```python
from build123d import *

# Parameters (mm, degrees)
SKETCH1_W      = 16
SKETCH1_H      = 16
EXTRUDE1_DEPTH = 240
SKETCH2_W      = 13
SKETCH2_H      = 13
EXTRUDE2_DEPTH = 242.064306773
SKETCH3_R      = 4
SKETCH3_R_2    = 1.85
EXTRUDE3_DEPTH = 242.064306773
SKETCH4_R      = 4
SKETCH4_R_2    = 1.85
EXTRUDE4_DEPTH = 242.064306773
FILLET1_R      = 1


with BuildPart() as part:
    # Sketch1 → Extrude1 (new body)
    with BuildSketch(Plane.XY):
        with Locations((8, 8)):
            Rectangle(SKETCH1_W, SKETCH1_H)
    extrude(amount=-EXTRUDE1_DEPTH)

    # Sketch2 → Extrude2 (cut, through all)
    with BuildSketch(Plane.XY):
        with Locations((8, 8)):
            Rectangle(SKETCH2_W, SKETCH2_H)
    extrude(amount=-EXTRUDE2_DEPTH, mode=Mode.SUBTRACT)

    # Sketch3 → Extrude3 (cut, through all)
    with BuildSketch(Plane(origin=(0, 16, 0), x_dir=(1, 0, 0), z_dir=(0, 1, 0))):
        with Locations(Location((8, 64, 0), (0, 0, 270))):
            Circle(SKETCH3_R)
        with Locations(Location((8, 32, 0), (0, 0, 270))):
            Circle(SKETCH3_R)
        with Locations((8, 0)):
            Circle(SKETCH3_R)
        with Locations(Location((8, 96, 0), (0, 0, 270))):
            Circle(SKETCH3_R)
        with Locations(Location((8, 128, 0), (0, 0, 270))):
            Circle(SKETCH3_R)
        with Locations(Location((8, 160, 0), (0, 0, 270))):
            Circle(SKETCH3_R)
        with Locations(Location((8, 192, 0), (0, 0, 270))):
            Circle(SKETCH3_R)
        with Locations(Location((8, 224, 0), (0, 0, 270))):
            Circle(SKETCH3_R)
        with Locations((8, 256)):
            Circle(SKETCH3_R)
        with Locations(Location((8, 48, 0), (0, 0, 270))):
            Circle(SKETCH3_R)
        with Locations(Location((8, 56, 0), (0, 0, 270))):
            Circle(SKETCH3_R_2)
        with Locations(Location((8, 40, 0), (0, 0, 270))):
            Circle(SKETCH3_R_2)
        with Locations(Location((8, 80, 0), (0, 0, 270))):
            Circle(SKETCH3_R)
        with Locations(Location((8, 88, 0), (0, 0, 270))):
            Circle(SKETCH3_R_2)
        with Locations(Location((8, 72, 0), (0, 0, 270))):
            Circle(SKETCH3_R_2)
        with Locations(Location((8, 16, 0), (0, 0, 270))):
            Circle(SKETCH3_R)
        with Locations(Location((8, 24, 0), (0, 0, 270))):
            Circle(SKETCH3_R_2)
        with Locations(Location((8, 8, 0), (0, 0, 270))):
            Circle(SKETCH3_R_2)
        with Locations(Location((8, 112, 0), (0, 0, 270))):
            Circle(SKETCH3_R)
        with Locations(Location((8, 120, 0), (0, 0, 270))):
            Circle(SKETCH3_R_2)
        with Locations(Location((8, 104, 0), (0, 0, 270))):
            Circle(SKETCH3_R_2)
        with Locations(Location((8, 144, 0), (0, 0, 270))):
            Circle(SKETCH3_R)
        with Locations(Location((8, 152, 0), (0, 0, 270))):
            Circle(SKETCH3_R_2)
        with Locations(Location((8, 136, 0), (0, 0, 270))):
            Circle(SKETCH3_R_2)
        with Locations(Location((8, 176, 0), (0, 0, 270))):
            Circle(SKETCH3_R)
        with Locations(Location((8, 184, 0), (0, 0, 270))):
            Circle(SKETCH3_R_2)
        with Locations(Location((8, 168, 0), (0, 0, 270))):
            Circle(SKETCH3_R_2)
        with Locations(Location((8, 208, 0), (0, 0, 270))):
            Circle(SKETCH3_R)
        with Locations(Location((8, 216, 0), (0, 0, 270))):
            Circle(SKETCH3_R_2)
        with Locations(Location((8, 200, 0), (0, 0, 270))):
            Circle(SKETCH3_R_2)
        with Locations((8, 240)):
            Circle(SKETCH3_R)
        with Locations((8, 248)):
            Circle(SKETCH3_R_2)
        with Locations(Location((8, 232, 0), (0, 0, 270))):
            Circle(SKETCH3_R_2)
    extrude(amount=-EXTRUDE3_DEPTH, mode=Mode.SUBTRACT)

    # Sketch4 → Extrude4 (cut, through all)
    with BuildSketch(Plane(origin=(16, 0, 0), x_dir=(0, 0, -1), z_dir=(1, 0, 0))):
        with Locations(Location((32, 8, 0), (0, 0, 90))):
            Circle(SKETCH4_R)
        with Locations(Location((64, 8, 0), (0, 0, 90))):
            Circle(SKETCH4_R)
        with Locations((0, 8)):
            Circle(SKETCH4_R)
        with Locations(Location((96, 8, 0), (0, 0, 90))):
            Circle(SKETCH4_R)
        with Locations(Location((128, 8, 0), (0, 0, 90))):
            Circle(SKETCH4_R)
        with Locations(Location((160, 8, 0), (0, 0, 90))):
            Circle(SKETCH4_R)
        with Locations(Location((192, 8, 0), (0, 0, 90))):
            Circle(SKETCH4_R)
        with Locations(Location((224, 8, 0), (0, 0, 90))):
            Circle(SKETCH4_R)
        with Locations((256, 8)):
            Circle(SKETCH4_R)
        with Locations(Location((48, 8.074203, 0), (0, 0, 90))):
            Circle(SKETCH4_R)
        with Locations(Location((40, 8.074203, 0), (0, 0, 90))):
            Circle(SKETCH4_R_2)
        with Locations(Location((56, 8.074203, 0), (0, 0, 90))):
            Circle(SKETCH4_R_2)
        with Locations(Location((80, 8, 0), (0, 0, 90))):
            Circle(SKETCH4_R)
        with Locations(Location((72, 8, 0), (0, 0, 90))):
            Circle(SKETCH4_R_2)
        with Locations(Location((88, 8, 0), (0, 0, 90))):
            Circle(SKETCH4_R_2)
        with Locations(Location((16, 8, 0), (0, 0, 90))):
            Circle(SKETCH4_R)
        with Locations(Location((8, 8, 0), (0, 0, 90))):
            Circle(SKETCH4_R_2)
        with Locations(Location((24, 8, 0), (0, 0, 90))):
            Circle(SKETCH4_R_2)
        with Locations(Location((112, 8, 0), (0, 0, 90))):
            Circle(SKETCH4_R)
        with Locations(Location((104, 8, 0), (0, 0, 90))):
            Circle(SKETCH4_R_2)
        with Locations(Location((120, 8, 0), (0, 0, 90))):
            Circle(SKETCH4_R_2)
        with Locations(Location((144, 8, 0), (0, 0, 90))):
            Circle(SKETCH4_R)
        with Locations(Location((136, 8, 0), (0, 0, 90))):
            Circle(SKETCH4_R_2)
        with Locations(Location((152, 8, 0), (0, 0, 90))):
            Circle(SKETCH4_R_2)
        with Locations(Location((176, 8, 0), (0, 0, 90))):
            Circle(SKETCH4_R)
        with Locations(Location((168, 8, 0), (0, 0, 90))):
            Circle(SKETCH4_R_2)
        with Locations(Location((184, 8, 0), (0, 0, 90))):
            Circle(SKETCH4_R_2)
        with Locations(Location((208, 8, 0), (0, 0, 90))):
            Circle(SKETCH4_R)
        with Locations(Location((200, 8, 0), (0, 0, 90))):
            Circle(SKETCH4_R_2)
        with Locations(Location((216, 8, 0), (0, 0, 90))):
            Circle(SKETCH4_R_2)
        with Locations((240, 8)):
            Circle(SKETCH4_R)
        with Locations(Location((232, 8, 0), (0, 0, 90))):
            Circle(SKETCH4_R_2)
        with Locations((248, 8)):
            Circle(SKETCH4_R_2)
    extrude(amount=-EXTRUDE4_DEPTH, mode=Mode.SUBTRACT)

    # Fillet1
    fillet1_edges = [part.edges().sort_by_distance(p)[0] for p in [
        (0, 16, -120),
        (16, 16, -120),
        (16, 0, -120),
        (0, 0, -120),
    ]]
    fillet(fillet1_edges, radius=FILLET1_R)


solid = part.part
```
Geometry check sheet. Reference: the model listing, model coordinates, mm. A direction names the side the tool comes from. Coordinates: 2 decimals unless noted, no trailing zeros. Write each loop counter-clockwise with the first axis right and the second up, starting at its lowest first coordinate (ties: lowest second). Pieces come first, ordered by that corner, then holes. Notation, with made-up numbers: M 8.5,-17 L 47.5,-17 A30 ccw 47.5,10 Z; hole C 46,78.25 d1. An arc over 180 degrees is marked long. One line per item, written item: value. Start each with the question number.
(1) Sectioned sample at A-A, the plane z = -208. Enter the section's corners in (x, y).
(2) Depth check by flat-ended pin: pin 1 (2 mm diameter, centred on y = 8, z = -200, fed in from -X). Enter the tip coordinate at first touch or a pass-through.
(3) Release check for a two-part mould opening along Z. For faces 3 (the face through (6, 0, -118)), 4 (the face through (0.761, 7.599, -73.806)), 5 (the face through (15, 2, 0)) record: released by +Z, released by -Z, zero draft, split by the parting line, or undercut.
(4) Sectioned sample at B-B, the plane z = -78. Enter the section's corners in (x, y).
(5) Tool access check on faces 1 (the face through (6, 14.5, -118)), 2 (the face through (8, 1, -116)). Record the directions out of +Z, -Z, +X, -X, +Y, -Y that give a thin tool (end or side, any length) a straight path to the whole face; none if there is none.
(6) Scan lines: line 1 along X through (y, z) = (9.5, -133.5); line 2 along X through (y, z) = (0.9, -72). Record each from-to range of solid material in increasing order. Write a range as [from, to].
Filled sheet:
1. outline: M 0,1 A1 ccw 1,0 L 4,0 L 4,1.5 L 1.5,1.5 L 1.5,4 L 0,4 Z; M 0,12 L 1.5,12 L 1.5,14.5 L 4,14.5 L 4,16 L 1,16 A1 ccw 0,15 Z; M 12,0 L 15,0 A1 ccw 16,1 L 16,4 L 14.5,4 L 14.5,1.5 L 12,1.5 Z; M 12,14.5 L 14.5,14.5 L 14.5,12 L 16,12 L 16,15 A1 ccw 15,16 L 12,16 Z
2. pin 1: through
3. face 3: zero draft
3. face 4: undercut
3. face 5: released by +Z
4. outline: M 0,1 A1 ccw 1,0 L 4.54,0 L 4.54,1.5 L 1.5,1.5 L 1.5,4.54 L 0,4.54 Z; M 0,11.46 L 1.5,11.46 L 1.5,14.5 L 4.54,14.5 L 4.54,16 L 1,16 A1 ccw 0,15 Z; M 11.46,0 L 15,0 A1 ccw 16,1 L 16,4.54 L 14.5,4.54 L 14.5,1.5 L 11.46,1.5 Z; M 11.46,14.5 L 14.5,14.5 L 14.5,11.46 L 16,11.46 L 16,15 A1 ccw 15,16 L 11.46,16 Z
5. face 1: +Z, -Z
5. face 2: +Y, -Y
6. line 1: [0, 1.5], [14.5, 16]
6. line 2: [0.01, 6.15], [9.85, 15.99]
